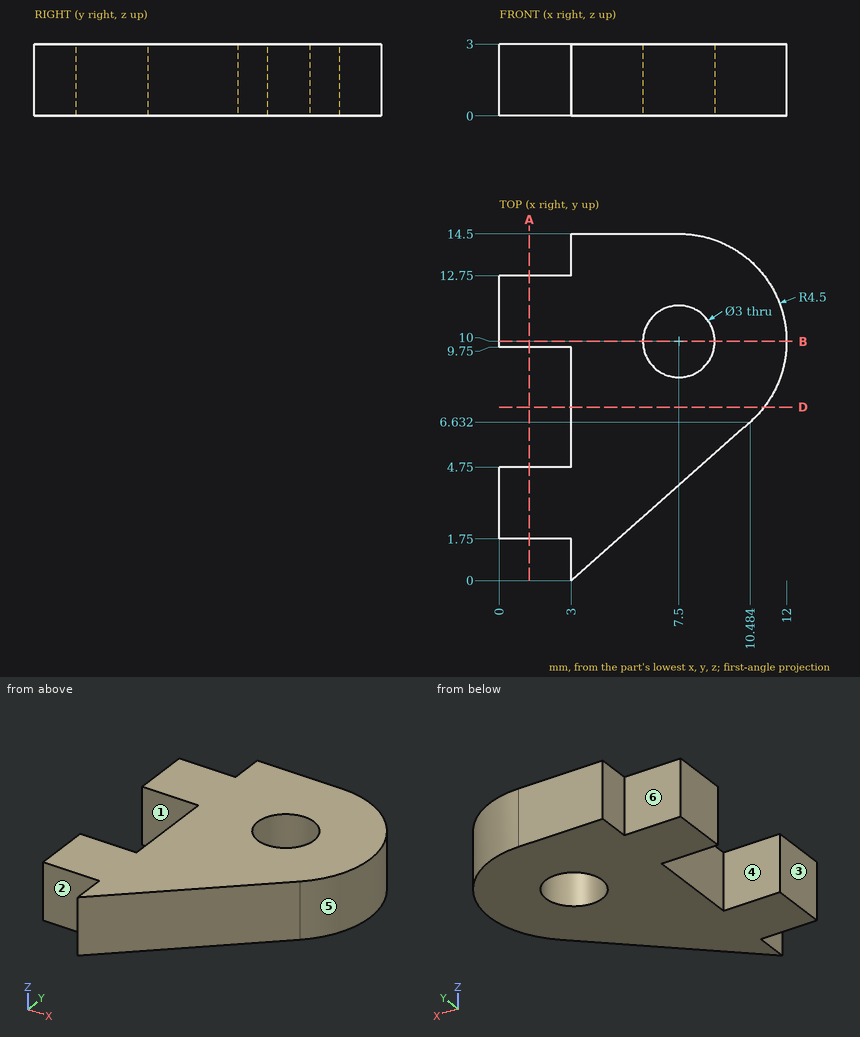
Verification items for this drawing (mm, ordinates from the low corner). A direction names the side the tool comes from. Give positions to 0.01 mm unless a question says otherwise; leave off trailing zeros. Write each loop counter-clockwise with the first axis right and the second up, starting at its lowest first coordinate (ties: lowest second). Pieces come first, ordered by that corner, then holes. Notation, with made-up numbers: (52.5, 34) -> (63.5, 34) arc R18 ccw to (63.5, 40) -> close; hole circle Ø2 at (29, 22.25). An arc over 180 degrees is marked (long way). Use CSV: the item, a comma, the result in double quotes. Start each with the question number.
Q1. Depth check by flat-ended pin: P1, Ø1.5, axis at x = 1, z = 1.5, coming from the +Y side; P2, Ø0.9, axis at y = 8, z = 2, coming from the -X side; P3, Ø1.8, axis at x = 7.5, y = 10, coming from the -Z side; P4, Ø1, axis at y = 3.5, z = 1.5, coming from the +X side (1 decimal). Enter the tip coordinate at first touch or a pass-through.
Q2. Release check for a two-part mould opening along Y. For the marked faces 1, 2 and 3 record: +Y half, -Y half, draft (parallel to the pull), parting line (faces both ways), or undercut.
Q3. Cross-section at B-B on y = 10. Enter the section's corners in (x, z), and give its area (3 significant figures).
Q4. Cross-section at D-D on y = 7.25. Enter the section's corners in (x, z).
Q5. Tool access check on the marked faces 4, 5 and 6. Record the directions out of +Z, -Z, +X, -X, +Y, -Y that give a thin tool (end or side, any length) a straight path to the whole face; none if there is none.
Q6. Cross-section at A-A on x = 1.25. Enter the section's corners in (y, z), and give its area (3 significant figures).
Q7. Scan lines: line 1 along Y through (x, z) = (1.25, 2.4); line 2 along Y through (x, z) = (7.5, 1.05); line 3 along X through (y, z) = (5, 1.95) (1 decimal). Record each from-to range of solid material in increasing order.
Working result:
1,P1,"stops at y = 12.75"
1,P2,"stops at x = 3"
1,P3,"passes through"
1,P4,"stops at x = 7.5"
2,face 1,"undercut"
2,face 2,"-Y half"
2,face 3,"draft"
3,outline,"(0, 0) -> (6, 0) -> (6, 3) -> (0, 3) -> close; (9, 0) -> (12, 0) -> (12, 3) -> (9, 3) -> close"
3,area,"27.0 mm^2"
4,outline,"(3, 0) -> (11.06, 0) -> (11.06, 3) -> (3, 3) -> close"
5,face 4,"+Z, -Z, -X"
5,face 5,"+Z, -Z, +X"
5,face 6,"+Z, -Z, -X, +Y"
6,outline,"(1.75, 0) -> (4.75, 0) -> (4.75, 3) -> (1.75, 3) -> close; (9.75, 0) -> (12.75, 0) -> (12.75, 3) -> (9.75, 3) -> close"
6,area,"18.0 mm^2"
7,line 1,"y = 1.75 to 4.75, 9.75 to 12.75"
7,line 2,"y = 3.99 to 8.5, 11.5 to 14.5"
7,line 3,"x = 3 to 8.6"
